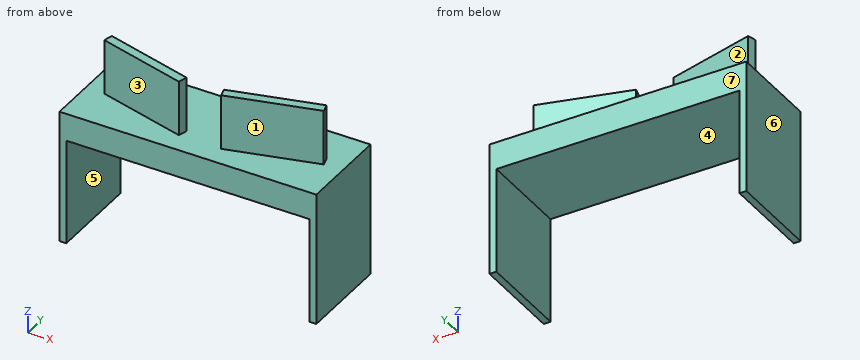
```python
from build123d import *

# Parameters (mm, degrees)
F0_W     = 38.1
F0_H     = 508
F1_DEPTH = 584.2
F2_W     = 1384.3
F2_H     = 508
F2_W_2   = 38.1
F3_DEPTH = 152.4
F5_DEPTH = 304.8


with BuildPart() as f1:
    # F0 (on Top) → F1 (new body)
    with BuildSketch(Plane.XY):
        with Locations((19.05, 254)):
            Rectangle(F0_W, F0_H)
        with Locations((1403.35, 254)):
            Rectangle(F0_W, F0_H)
    extrude(amount=F1_DEPTH)

    # F2 (on face) → F3 (join)
    with BuildSketch(Plane.XY.offset(584.2)):
        with Locations((730.25, 254)):
            Rectangle(F2_W, F2_H)
        with Locations((19.05, 254)):
            Rectangle(F2_W_2, F2_H)
    extrude(amount=F3_DEPTH)

    # F4 (on face) → F5 (join)
    with BuildSketch(Plane.XY.offset(736.6)):
        Polygon((594.371156, 112.925447), (607.519164, 161.994479), (116.828844, 293.474553), (103.680836, 244.405521), align=None)
        Polygon((1318.719164, 244.405521), (1305.571156, 293.474553), (814.880836, 161.994479), (828.028844, 112.925447), align=None)
    extrude(amount=F5_DEPTH)


solid = f1.part
```
Can you work these out from the model? Positions are in its coordinate system, mm. Face numbers are marked on the shaded views. A direction names the side the tool comes from. Coordinates: 2 decimals unless noted, no trailing zeros. Order: outer loops, then holes, each group sorted by start corner. A loop starts at its lowest first (then second) coordinate and runs counter-clockwise, first axis right, second up.
1. If we section it at A-A (z = 881.5): Please give me the cut outline in (x, y), then the cut area to 3 significant figures.
2. If we section it at D-D (z = 228.5): Please give me the cut outline in (x, y).
3. Thinking about a two-plate mould opening in X: for the marked faces 5, 6 and 7, which applies, +X half, -X half, draft (parallel to the pull), parting line (faces both ways), or undercut?
4. If we section it at B-B (y = 72.5): Please give me the cut outline in (x, z).
5. If we section it at C-C (x = 527): Please give me the cut outline in (y, z).
6. I need wall thicknesses on line 1 (X direction, y = 368.5, z = 252.5); line 2 (Z direction, x = 232, y = 37); line 3 (Y direction, x = 1255, z = 809.5). Which ranges of each line are inside material? Lowest first, please.
7. I'm going to push flat-ended pins straight in: pin 1 (4 mm diameter, centred on x = 1225, y = 95.5, fed in from +Z); pin 2 (2 mm diameter, centred on x = 689, y = 451, fed in from -Z). Where does each tip first touch, or does it pass through?
8. For the marked faces 1, 2, 3 and 4, which set-ups out of +Z, -Z, +X, -X, +Y, -Y let a thin tool reach every point of the face, with its end or its side?
Entries:
1. outline: (103.68, 244.41) - (594.37, 112.93) - (607.52, 161.99) - (116.83, 293.47) - close; (814.88, 161.99) - (828.03, 112.93) - (1318.72, 244.41) - (1305.57, 293.47) - close
1. area: 51,600 mm2
2. outline: (0, 0) - (38.1, 0) - (38.1, 508) - (0, 508) - close; (1384.3, 0) - (1422.4, 0) - (1422.4, 508) - (1384.3, 508) - close
3. face 5: undercut
3. face 6: -X half
3. face 7: draft
4. outline: (0, 0) - (38.1, 0) - (38.1, 584.2) - (1384.3, 584.2) - (1384.3, 0) - (1422.4, 0) - (1422.4, 736.6) - (0, 736.6) - close
5. outline: (0, 584.2) - (508, 584.2) - (508, 736.6) - (183.57, 736.6) - (183.57, 1041.4) - (130.98, 1041.4) - (130.98, 736.6) - (0, 736.6) - close
6. line 1: x = 0 to 38.1, 1384.3 to 1422.4
6. line 2: z = 584.2 to 736.6
6. line 3: y = 227.33 to 279.92
7. pin 1: stops at z = 736.6
7. pin 2: stops at z = 584.2
8. face 1: +Z, +X, -Y
8. face 2: +Z, +Y
8. face 3: +Z, -X, -Y
8. face 4: -Z, +Y, -Y
